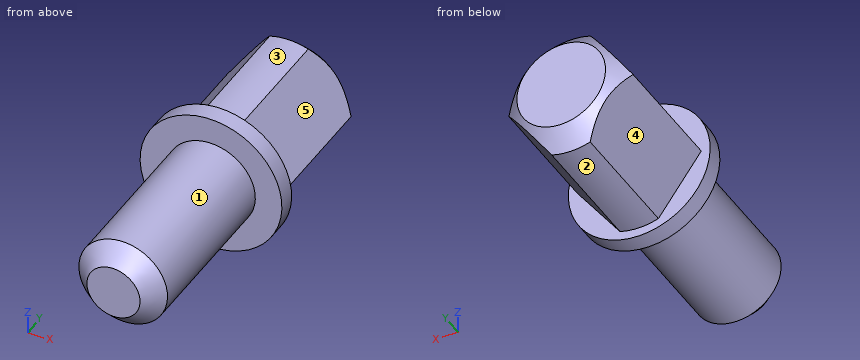
```python
from build123d import *

# Parameters (mm, degrees)
SKETCH_2_R          = 6.282667793
CUT_EXTRUDE_2_DEPTH = 8


with BuildPart() as part:
    # 草图1 → 旋转1 (revolve)
    with BuildSketch(Plane.XY, mode=Mode.PRIVATE) as revolve_1_sk:
        Polygon((0, 0), (0, 19), (2.5, 19), (3.5, 18), (3.5, 11), (4, 11), (4, 10), (2.5, 10), (2.5, 1), (1.5, 0), align=None)
    revolve(revolve_1_sk.sketch.rotate(Axis((0, 0, 0), (0, 1, 0)), 90), axis=Axis((0, 0, 0), (0, 1, 0)))

    # 草图2 → 切除-拉伸2 (cut)
    with BuildSketch(Plane(origin=(0, 19, 0), x_dir=(1, 0, 0), z_dir=(0, 1, 0))):
        Circle(SKETCH_2_R)
        Polygon((0, 4.820824702), (-3.5, 0), (0, -4.820824702), (3.5, 0), align=None, mode=Mode.SUBTRACT)
    extrude(amount=-CUT_EXTRUDE_2_DEPTH, mode=Mode.SUBTRACT)


solid = part.part
```
For this review, take the finished solid that the model builds, in its own axes (mm). Face numbers are marked on the shaded views. A direction names the side the tool comes from. Coordinates: 2 decimals unless noted, no trailing zeros. Loops run counter-clockwise (first coordinate to the right, second up) from the corner with the lowest first, then second, coordinate; pieces in that order, holes last.
1. For the marked faces 1, 2, 3, 4 and 5, list the 3-axis set-ups (+Z, -Z, +X, -X, +Y, -Y) from which the entire face can be reached by the end or side of a thin tool; tool diameter is ignored.
2. For line 1 (Z direction, x = 2.25, y = 6.75); line 2 (Y direction, x = -2.75, z = -1.75); line 3 (X direction, y = 13.75, z = 2.75), list the stretches that pass through material, from the lowest coordinate up.
3. Add section D-D, the plane y = 4.75. Give the boundary of the cut face in (x, z).
4. Insertion check: P1, Ø1.5, axis at x = -2, y = 11.5, coming from the -Z side; P2, Ø4, axis at x = 0, y = 15, coming from the +Z side; P3, Ø4, axis at y = 15.5, z = 0.5, coming from the +X side. Each pin has a flat end and moves straight along its axis. Give the tip position at first contact, or say it passes through.
5. Add section A-A, the plane x = 0. Give the boundary of the cut face in (y, z), then the cut area to 3 significant figures.
6. Add section B-B, the plane y = 11.75. Give the boundary of the cut face in (x, z).
7. Add section C-C, the plane z = 3.75. Give the boundary of the cut face in (x, y), then the cut area to 3 significant figures.
Result:
1. face 1: -Y
1. face 2: -Z, +Y
1. face 3: +Z, +Y
1. face 4: -Z, -X, +Y
1. face 5: +Z, +X, +Y
2. line 1: z = -1.09 to 1.09
2. line 2: y = 10 to 11
2. line 3: x = -1.5 to 1.5
3. outline: circle Ø5 at (0, 0)
4. P1: stops at z = -3.73
4. P2: stops at z = 3.5
4. P3: stops at x = 3.5
5. outline: (0, -1.5) - (1, -2.5) - (10, -2.5) - (10, -4) - (11, -4) - (11, -3.5) - (18, -3.5) - (19, -2.5) - (19, 2.5) - (18, 3.5) - (11, 3.5) - (11, 4) - (10, 4) - (10, 2.5) - (1, 2.5) - (0, 1.5) - close
5. area: 112 mm2
6. outline: (-3.5, 0) - (-1.08, -3.33) arc R3.5 ccw to (1.08, -3.33) - (3.5, 0) - (1.08, 3.33) arc R3.5 ccw to (-1.08, 3.33) - close
7. outline: (-1.39, 10) - (1.39, 10) - (1.39, 11) - (-1.39, 11) - close
7. area: 2.78 mm2
